from build123d import *

# Parameters (mm, degrees)
SKETCH1_R           = 1.651
BOSS_EXTRUDE1_DEPTH = 1.5875


with BuildPart() as part:
    # Sketch1 → Boss-Extrude1 (new body)
    with BuildSketch(Plane(origin=(0, 0, 0), x_dir=(-1, 0, 0), z_dir=(0, 0, -1))):
        with BuildLine():
            Line((-129.38125, 0), (129.38125, 0))
            ThreePointArc((129.38125, 0), (133.310112053, 1.627387947), (134.9375, 5.55625))
            Line((134.9375, 5.55625), (134.9375, 53.373846086))
            ThreePointArc((134.9375, 53.373846086), (134.905262076, 53.971512085), (134.8089224, 54.562242647))
            Line((134.8089224, 54.562242647), (122.750794586, 109.634404323))
            ThreePointArc((122.750794586, 109.634404323), (122.197927005, 111.112127049), (121.251984239, 112.374869817))
            Line((121.251984239, 112.374869817), (85.387369836, 148.239484219))
            ThreePointArc((85.387369836, 148.239484219), (84.124627068, 149.185426985), (82.646904343, 149.738294567))
            Line((82.646904343, 149.738294567), (27.574742607, 161.796422401))
            ThreePointArc((27.574742607, 161.796422401), (26.984012045, 161.892762078), (26.386346045, 161.925000002))
            Line((26.386346045, 161.925000002), (-26.386346022, 161.925000002))
            ThreePointArc((-26.386346022, 161.925000002), (-26.984012021, 161.892762078), (-27.574742583, 161.796422402))
            Line((-27.574742583, 161.796422402), (-82.646904321, 149.738294575))
            ThreePointArc((-82.646904321, 149.738294575), (-84.124627046, 149.185426993), (-85.387369815, 148.239484227))
            Line((-85.387369815, 148.239484227), (-121.251984217, 112.374869825))
            ThreePointArc((-121.251984217, 112.374869825), (-122.197926983, 111.112127057), (-122.750794565, 109.634404332))
            Line((-122.750794565, 109.634404332), (-134.808922399, 54.562242596))
            ThreePointArc((-134.808922399, 54.562242596), (-134.905262076, 53.971512033), (-134.9375, 53.373846033))
            Line((-134.9375, 53.373846033), (-134.9375, 5.55625))
            ThreePointArc((-134.9375, 5.55625), (-133.310112053, 1.627387947), (-129.38125, 0))
        make_face()
        with Locations((-53.975, 26.9875)):
            Circle(SKETCH1_R, mode=Mode.SUBTRACT)
        with Locations((53.975, 26.9875)):
            Circle(SKETCH1_R, mode=Mode.SUBTRACT)
        with Locations((46.070544257, 73.058044257)):
            Circle(SKETCH1_R, mode=Mode.SUBTRACT)
        with Locations((84.236632771, 111.224132771)):
            Circle(SKETCH1_R, mode=Mode.SUBTRACT)
        with Locations((-46.070544257, 73.058044257)):
            Circle(SKETCH1_R, mode=Mode.SUBTRACT)
        with Locations((-84.236632771, 111.224132771)):
            Circle(SKETCH1_R, mode=Mode.SUBTRACT)
        with Locations((-107.95, 26.9875)):
            Circle(SKETCH1_R, mode=Mode.SUBTRACT)
        with Locations((107.95, 26.9875)):
            Circle(SKETCH1_R, mode=Mode.SUBTRACT)
        with Locations((0, 80.9625)):
            Circle(SKETCH1_R, mode=Mode.SUBTRACT)
        with Locations((0, 134.9375)):
            Circle(SKETCH1_R, mode=Mode.SUBTRACT)
        with Locations((0, 26.9875)):
            Circle(SKETCH1_R, mode=Mode.SUBTRACT)
    extrude(amount=-BOSS_EXTRUDE1_DEPTH)


solid = part.part
CAD build for the part. Positions are in the model's coordinates, mm. Round coordinates to 2 decimals unless told otherwise and drop trailing zeros. Loops run counter-clockwise (first coordinate to the right, second up) from the corner with the lowest first, then second, coordinate; pieces in that order, holes last. Notation, with made-up numbers: (60, -22) - (74, -22) arc R18 ccw to (74, -8) - close; hole circle Ø4 at (56, 85). An arc over 180 degrees is marked (long way). Put each result on its own line as item: value.
1. Pin check, flat tip, straight feed: P1, Ø2.5, axis at x = 53.98, y = 26.99, coming from the -Z side (3 decimals). Stop position of the tip, or through.
Geometry check:
P1: through
2. Slice it at B-B on y = 128. List the corners of the cut face in (x, z).
Geometry check:
outline: (-105.63, 0) - (105.63, 0) - (105.63, 1.59) - (-105.63, 1.59) - close
3. Wall check: line 1 (Y direction, x = 0, z = 0.4) (1 decimal); line 2 (X direction, y = 26, z = 0.55); line 3 (X direction, y = 53.5, z = 0.25). Give the ranges that are in metal, low to high.
Geometry check:
line 1: 0 to 25.3, 28.6 to 79.3, 82.6 to 133.3, 136.6 to 161.9
line 2: -134.94 to -109.27, -106.63 to -55.3, -52.65 to -1.32, 1.32 to 52.65, 55.3 to 106.63, 109.27 to 134.94
line 3: -134.94 to 134.94
4. Slice it at A-A on x = 89. List the corners of the cut face in (y, z).
Geometry check:
outline: (0, 0) - (144.63, 0) - (144.63, 1.59) - (0, 1.59) - close
